Solid Edge part; units mm, degrees
sketch "Sketch1" plane through (0, 0, 0) normal (0, 0, 1) x (1, 0, 0)
  circle A0 centre (-31.2598, 30.8498) radius 10
extrude "Protrusion1" add sketch "Sketch1" along normal blind 7.5
fillet "Round_1" radius 2 1 edges at (-41.2598, 30.8498, 7.5)
sketch "Sketch2" plane through (-31.2598, 30.8498, 0) normal (0, 0, -1) x (1, 0, 0)
  circle A0 centre (0, 0) radius 9
extrude "ExtrudedProtrusion_2" add sketch "Sketch2" along normal blind 1.5
sketch "Sketch3" plane through (-31.2598, 30.8498, 7.5) normal (0, 0, 1) x (1, 0, 0)
  circle A0 centre (0, 0) radius 2.5
extrude "ExtrudedProtrusion_3" add sketch "Sketch3" along normal blind 12.7
sketch "Sketch4" plane through (-31.2598, 30.8498, 7.5) normal (0, 0, 1) x (1, 0, 0)
  line L0 (1.819, 3.5694) -> (-1.811, 3.5694)
  line L1 (-3.8317, 0.0694) -> (-1.811, 3.5694)
  line L2 (-3.8317, 0.0694) -> (-1.811, -3.4306)
  line L3 (-1.811, -3.4306) -> (1.819, -3.4306)
  line L4 (3.8397, 0.0694) -> (1.819, -3.4306)
  line L5 (3.8397, 0.0694) -> (1.819, 3.5694)
extrude "ExtrudedProtrusion_4" add sketch "Sketch4" along normal blind 2
sketch "Sketch5" plane through (-31.2598, 30.8498, -1.5) normal (0, 0, -1) x (0, 1, 0)
  circle A0 centre (-3.3065, -6.4712) radius 1
  circle A1 centre (3.3276, -6.4738) radius 1
  circle A2 centre (-6.0923, -4.2376) radius 1
  circle A3 centre (5.9466, -4.3494) radius 1
  circle A4 centre (-0.002, -7.3079) radius 1
extrude "ExtrudedProtrusion_5" add sketch "Sketch5" along normal blind 1
sketch "Sketch6" plane through (-31.2598, 30.8498, 20.2) normal (0, 0, 1) x (1, 0, 0)
  line L0 (-1.6783, 1.9858) -> (1.6783, 1.9858)
extrude "Cutout1" cut sketch "Sketch6" against normal up to vertex (10.7 mm away) material side at (-31.2598, 32.8856, 20.2)
The listing builds one solid part. Answer for the finished solid, in the listing's coordinates (mm). A direction names the side the tool comes from. Give positions to 0.01 mm unless a question says otherwise; leave off trailing zeros. Loops run counter-clockwise (first coordinate to the right, second up) from the corner with the lowest first, then second, coordinate; pieces in that order, holes last. Notation, with made-up numbers: (72, 24.25) - (89, 24.25) arc R8 ccw to (89, 36.25) - close; hole circle Ø3 at (38.25, -21.75). An arc over 180 degrees is marked (long way). Answer as a JSON object with one key per item and string values.
1. Find the intervals of material crossed by L1, parallel to Z at x = -33.75, y = 38.25; L2, parallel to X at y = 26.5, z = 3.25; L3, parallel to Z at x = -31.25, y = 34, in increasing order. Write a range as [from, to].
Determined:
{"L1": "[-1.5, 7.5]", "L2": "[-40.26, -22.26]", "L3": "[-1.5, 9.5]"}
2. For faces 4 (the flat face through (-31, 34.419, 8)), 5 (the flat face through (-31, 27, 7.5)), 6 (the cylindrical face through (-36.755, 27.327, -1.993)), determine the directions among +Z, -Z, +X, -X, +Y, -Y from which every point of the face is accessible in a straight line to the end or side of a thin tool.
Determined:
{"face 4": "+Z, +X, -X, +Y", "face 5": "+Z", "face 6": "-Z"}
3. A cutting plane is placed at D-D (z = 2.75). Write down the section's boundary in (x, y).
Determined:
{"outline": "circle Ø20 at (-31.26, 30.85)"}
4. Flat-ended cylindrical pins translate along their axes: pin 1 Ø2 at (x, y) = (-25.5, 25.5) entering from -Z; pin 2 Ø5 at (x, y) = (-23.5, 30.5) entering from +Z; pin 3 Ø1.6 at (x, z) = (-31, 9) entering from -Y; pin 4 Ø9 at (x, y) = (-31.5, 26.5) entering from -Z. Find the tip coordinate at first contact, or state that the pin passes through.
Determined:
{"pin 1": "z = -1.5", "pin 2": "z = 7.5", "pin 3": "y = 27.42", "pin 4": "z = -2.5"}
5. For a pull along Y with two mould halves and no side action, classify faces 1 (the cylindrical face through (-38.034, 35.131, -1.993)), 2 (the flat face through (-31, 27.419, 8)), 3 (the flat face through (-34.1, 32.64, 8.49)) as pulls with the +Y half, pulls with the -Y half, needs draft (parallel to the pull), parting line crosses it, or undercut.
Determined:
{"face 1": "undercut", "face 2": "pulls with the -Y half", "face 3": "pulls with the +Y half"}
6. A cutting plane is placed at A-A (z = 9). Write down the section's boundary in (x, y).
Determined:
{"outline": "(-35.09, 30.92) - (-33.07, 27.42) - (-29.44, 27.42) - (-27.42, 30.92) - (-29.44, 34.42) - (-33.07, 34.42) - close"}
7. A cutting plane is placed at B-B (z = 18.5). Write down the section's boundary in (x, y).
Determined:
{"outline": "(-32.78, 32.84) arc R2.5 ccw (long way) to (-29.74, 32.84) - close"}
8. A cutting plane is placed at C-C (z = 6.5). Write down the section's boundary in (x, y).
Determined:
{"outline": "circle Ø19.46 at (-31.26, 30.85)"}
